from build123d import *
from OCP.BRepAlgoAPI import BRepAlgoAPI_Cut
from OCP.TopTools import TopTools_ListOfShape

# Parameters (mm, degrees)
SKETCH1_R           = 150
BOSS_EXTRUDE1_DEPTH = 50
SKETCH2_W           = 180
SKETCH2_H           = 150
BOSS_EXTRUDE2_DEPTH = 120
SKETCH4_W           = 150
SKETCH4_H           = 60
CUT_EXTRUDE1_DEPTH  = 180
BOSS_EXTRUDE3_DEPTH = 180
SKETCH5_W           = 102.267162736
SKETCH5_H           = 75
CUT_EXTRUDE3_DEPTH  = 180
CUT_EXTRUDE4_START  = 100
CUT_EXTRUDE4_DEPTH  = 100
CUT_EXTRUDE5_START  = -2.26716
CUT_EXTRUDE5_DEPTH  = 2.26716
SKETCH12_R          = 40
CUT_EXTRUDE6_DEPTH  = 20
CUT_EXTRUDE7_START  = -20
SKETCH11_R          = 40
CUT_EXTRUDE7_DEPTH  = 20
SKETCH15_W          = 102.26716
SKETCH15_H          = 60
CUT_EXTRUDE8_DEPTH  = 408
SKETCH16_R          = 250
BOSS_EXTRUDE4_DEPTH = 50


with BuildPart() as part:
    # Sketch1 → Boss-Extrude1 (new body)
    with BuildSketch(Plane(origin=(0, 0, 0), x_dir=(1, 0, 0), z_dir=(0, 1, 0))):
        with Locations(Location((0, 0, 0), (0, 0, 270))):
            Circle(SKETCH1_R)
    extrude(amount=BOSS_EXTRUDE1_DEPTH)

    # Sketch2 → Boss-Extrude2 (add)
    with BuildSketch(Plane(origin=(0, 50, 0), x_dir=(1, 0, 0), z_dir=(0, 1, 0))):
        Rectangle(SKETCH2_W, SKETCH2_H)
    extrude(amount=BOSS_EXTRUDE2_DEPTH)

    # Sketch4 → Cut-Extrude1 (cut)
    with BuildSketch(Plane.ZY.offset(90)):
        with Locations((0, 140)):
            Rectangle(SKETCH4_W, SKETCH4_H)
    extrude(amount=-CUT_EXTRUDE1_DEPTH, mode=Mode.SUBTRACT)

    # Sketch3 → Boss-Extrude3 (add)
    with BuildSketch(Plane(origin=(90, 0, 0), x_dir=(0, 0, -1), z_dir=(1, 0, 0))):
        with BuildLine():
            Line((-75, 110), (-75, 50))
            Line((-75, 50), (75, 50))
            Line((75, 50), (75, 110))
            ThreePointArc((75, 110), (0, 185), (-75, 110))
        make_face()
    extrude(amount=-BOSS_EXTRUDE3_DEPTH)

    # Sketch5 → Cut-Extrude3 (cut)
    with BuildSketch(Plane.XY.offset(75)):
        with Locations((0, 147.5)):
            Rectangle(SKETCH5_W, SKETCH5_H)
    extrude(amount=-CUT_EXTRUDE3_DEPTH, mode=Mode.SUBTRACT)

    # Sketch8 → Cut-Extrude4 (cut)
    with BuildSketch(Plane(origin=(-51.133581368, 0, 0), x_dir=(0, 0, -1), z_dir=(1, 0, 0)).offset(CUT_EXTRUDE4_START)):
        with BuildLine():
            Line((-75, 110), (75, 110))
            ThreePointArc((75, 110), (0, 35), (-75, 110))
        make_face()
    extrude(amount=-CUT_EXTRUDE4_DEPTH, mode=Mode.SUBTRACT)

    # Sketch10 → Cut-Extrude5 (cut)
    with BuildSketch(Plane.ZY.offset(-48.866418632).offset(CUT_EXTRUDE5_START)):
        with BuildLine():
            Line((-75, 110), (75, 110))
            ThreePointArc((75, 110), (0, 35), (-75, 110))
        make_face()
    extrude(amount=CUT_EXTRUDE5_DEPTH, mode=Mode.SUBTRACT)


with BuildPart() as cut_extrude6_tool:
    # Sketch12 → Cut-Extrude6 (new body)
    with BuildSketch(Plane.ZY.offset(-51.133581368)):
        with Locations((0, 110)):
            Circle(SKETCH12_R)
    extrude(amount=-CUT_EXTRUDE6_DEPTH)


with BuildPart() as part_1:
    add(part.part)

    # Cut-Extrude6: cut by cut_extrude6_tool, with a tolerance
    cut_extrude6_stock = TopTools_ListOfShape()
    cut_extrude6_stock.Append(part_1.part.wrapped)
    cut_extrude6_tools = TopTools_ListOfShape()
    cut_extrude6_tools.Append(cut_extrude6_tool.part.wrapped)
    cut_extrude6_cut = BRepAlgoAPI_Cut()
    cut_extrude6_cut.SetArguments(cut_extrude6_stock)
    cut_extrude6_cut.SetTools(cut_extrude6_tools)
    cut_extrude6_cut.SetFuzzyValue(0.00001)
    cut_extrude6_cut.Build()
    add(Compound.cast(cut_extrude6_cut.Shape()).solids(), mode=Mode.REPLACE)

    # Sketch11 → Cut-Extrude7 (cut)
    with BuildSketch(Plane(origin=(-51.133581368, 0, 0), x_dir=(0, 0, -1), z_dir=(1, 0, 0)).offset(CUT_EXTRUDE7_START)):
        with Locations(Location((0, 110, 0), (0, 0, 180))):
            Circle(SKETCH11_R)
    extrude(amount=CUT_EXTRUDE7_DEPTH, mode=Mode.SUBTRACT)

    # Sketch15 → Cut-Extrude8 (cut)
    with BuildSketch(Plane.XY.offset(75)):
        with Locations((-1.368e-06, 80)):
            Rectangle(SKETCH15_W, SKETCH15_H)
    extrude(amount=-CUT_EXTRUDE8_DEPTH, mode=Mode.SUBTRACT)

    # Sketch16 → Boss-Extrude4 (add)
    with BuildSketch(Plane.XZ):
        with Locations(Location((0, 0, 0), (0, 0, 270))):
            Circle(SKETCH16_R)
    extrude(amount=-BOSS_EXTRUDE4_DEPTH)


solid = part_1.part
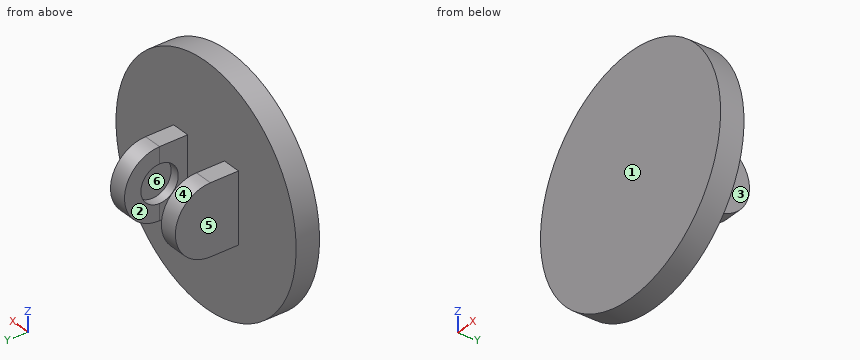
Design review of the part built by this model. Coordinates are the model's own, in mm. Face numbers are marked on the shaded views. A direction names the side the tool comes from. Coordinates: 2 decimals unless noted, no trailing zeros. Write each loop counter-clockwise with the first axis right and the second up, starting at its lowest first coordinate (ties: lowest second). Pieces come first, ordered by that corner, then holes. Notation, with made-up numbers: (-2, 52.25) - (49, 52.25) arc R17 cw to (49, 82.25) - close; hole circle Ø10 at (-39.75, 87.5). An arc over 180 degrees is marked (long way). One line per item, written item: value.
1) Add section B-B (y = 77). State the section outline as (x, z) points, plus the area to 3 significant figures.
Answer sheet:
outline: (-90, -75) - (-51.13, -75) - (-51.13, -22.61) - (-71.13, -22.61) - (-71.13, 22.61) - (-51.13, 22.61) - (-51.13, 75) - (-90, 75) - close; (51.13, -75) - (90, -75) - (90, 75) - (51.13, 75) - (51.13, 22.61) - (71.13, 22.61) - (71.13, -22.61) - (51.13, -22.61) - close
area: 9,850 mm2
2) To check wall thickness, follow probe 1 along Y at (x, z) = (-66, 0); probe 2 along X at (y, z) = (75, 48.5); probe 3 along X at (y, z) = (124.5, 34.5). State the ranges of each line that lie inside material, in increasing order.
Answer sheet:
probe 1: y = 0 to 70, 150 to 185
probe 2: x = -90 to -51.13, 51.13 to 90
probe 3: x = -90 to -71.13, 71.13 to 90
3) For the marked faces 1, 2 and 3, list the 3-axis set-ups (+Z, -Z, +X, -X, +Y, -Y) from which the entire face can be reached by the end or side of a thin tool; tool diameter is ignored.
Answer sheet:
face 1: +Z, -Z, +X, -X, -Y
face 2: +Z, -Z, +Y
face 3: +Z, -Z, +X, +Y
4) Mouldability with a two-part tool opening along X and no side actions: class the marked faces 4, 5 and 6 as +X half, -X half, draft (parallel to the pull), parting line (faces both ways), or undercut.
Answer sheet:
face 4: draft
face 5: -X half
face 6: undercut
5) Add section D-D (y = 174.5). State the section outline as (x, z) points.
Answer sheet:
outline: (-90, -38.27) - (-51.13, -38.27) - (-51.13, 38.27) - (-90, 38.27) - close; (51.13, -38.27) - (90, -38.27) - (90, 38.27) - (51.13, 38.27) - close
6) Insertion check: pin 1 (11.5 mm diameter, centred on x = 73.5, y = 74, fed in from -Z); pin 2 (19.5 mm diameter, centred on x = 63, y = 77, fed in from +Z); pin 3 (24 mm diameter, centred on y = 129.5, z = 13.5, fed in from -X); pin 4 (1 mm diameter, centred on x = 18.5, z = -192, fed in from -Y). Each pin has a flat end and moves straight along its axis. Give the tip position at first contact, or say it passes through.
Answer sheet:
pin 1: stops at z = -75
pin 2: stops at z = 75
pin 3: stops at x = -90
pin 4: stops at y = 0
7) Add section C-C (x = 0). State the section outline as (y, z) points.
Answer sheet:
outline: (0, -250) - (50, -250) - (50, 250) - (0, 250) - close
8) Add section A-A (z = 0). State the section outline as (x, y) points.
Answer sheet:
outline: (-250, 0) - (250, 0) - (250, 50) - (90, 50) - (90, 185) - (51.13, 185) - (51.13, 150) - (71.13, 150) - (71.13, 70) - (51.13, 70) - (51.13, 50) - (-51.13, 50) - (-51.13, 70) - (-71.13, 70) - (-71.13, 150) - (-51.13, 150) - (-51.13, 185) - (-90, 185) - (-90, 50) - (-250, 50) - close
